```python
from build123d import *

# Parameters (mm, degrees)
F1_DEPTH = 2.2
F3_DEPTH = 3


with BuildPart() as f1:
    # F0 (on Front) → F1 (new body)
    with BuildSketch(Plane.XZ):
        with BuildLine():
            Line((12.5, -9.5), (12.5, 9.5))
            Line((12.5, 9.5), (3.2765988609, 9.5))
            Line((3.2765988609, 9.5), (3.2765988609, 0.1127291822))
            ThreePointArc((3.2765988609, 0.1127291822), (0.0399120355, -3.3998448003), (-3.3149907831, 0))
            Line((-3.3149907831, 0), (-3.3149907831, 9.5))
            Line((-3.3149907831, 9.5), (-12.5, 9.5))
            Line((-12.5, 9.5), (-12.5, -9.5))
            Line((-12.5, -9.5), (12.5, -9.5))
        make_face()
    extrude(amount=F1_DEPTH)

    # F2 (on face) → F3 (join)
    with BuildSketch(Plane.XZ.offset(2.2)):
        with BuildLine():
            ThreePointArc((4.6765988609, 0.1539773139), (0.0605272986, -4.799695782), (-4.7154452944, 0))
            Line((-4.7154452944, 0), (-4.7154452944, 9.5))
            Line((-4.7154452944, 9.5), (-12.5, 9.5))
            Line((-12.5, 9.5), (-12.5, -9.5))
            Line((-12.5, -9.5), (12.5, -9.5))
            Line((12.5, -9.5), (12.5, 9.5))
            Line((12.5, 9.5), (4.6765988609, 9.5))
            Line((4.6765988609, 9.5), (4.6765988609, 0.1539773139))
        make_face()
    extrude(amount=F3_DEPTH)


solid = f1.part
```
The model under review builds one solid part; all positions refer to its coordinate system, in mm. A direction names the side the tool comes from. Round coordinates to 2 decimals unless told otherwise and drop trailing zeros. Write each loop counter-clockwise with the first axis right and the second up, starting at its lowest first coordinate (ties: lowest second). Pieces come first, ordered by that corner, then holes. Notation, with made-up numbers: (59, 76) - (99, 76) arc R19 ccw to (99, 106) - close; hole circle Ø2 at (-10, 28). An arc over 180 degrees is marked (long way). One line per question, with ' | ' between items.
Item 1: The part is to be moulded in two halves that separate along X. For faces 1 (the face through (0, -3, -9.5)), 2 (the face through (-12.5, -3, 0)), 3 (the face through (4.677, -4, 5)), 4 (the face through (-4, -2.2, 1)), say which applies: pulls with the +X half, pulls with the -X half, needs draft (parallel to the pull), parting line crosses it, or undercut.
Resolved:
face 1: needs draft | face 2: pulls with the -X half | face 3: undercut | face 4: undercut
Item 2: Add section C-C, the plane z = -0.75. Give the boundary of the cut face in (x, y).
Resolved:
outline: (-12.5, -5.2) - (-4.67, -5.2) - (-4.67, -2.2) - (-3.25, -2.2) - (-3.25, 0) - (-12.5, 0) - close; (3.22, -2.2) - (4.64, -2.2) - (4.64, -5.2) - (12.5, -5.2) - (12.5, 0) - (3.22, 0) - close
Item 3: To check wall thickness, follow probe 1 along X at (y, z) = (-1.7, 0) (3 decimals); probe 2 along X at (y, z) = (-3.2, 4.25); probe 3 along Y at (x, z) = (-3.75, 4.5). State the ranges of each line that lie inside material, in increasing order.
Resolved:
probe 1: x = -12.5 to -3.315, 3.282 to 12.5 | probe 2: x = -12.5 to -4.72, 4.68 to 12.5 | probe 3: y = -2.2 to 0
Item 4: Add section D-D, the plane y = -3.55. Give the boundary of the cut face in (x, z), then the cut area to 3 significant figures.
Resolved:
outline: (-12.5, -9.5) - (12.5, -9.5) - (12.5, 9.5) - (4.68, 9.5) - (4.68, 0.15) arc R4.7 cw (long way) to (-4.72, 0) - (-4.72, 9.5) - (-12.5, 9.5) - close | area: 350 mm2
Item 5: Add section B-B, the plane y = -1.5. Give the boundary of the cut face in (x, z) (3 decimals).
Resolved:
outline: (-12.5, -9.5) - (12.5, -9.5) - (12.5, 9.5) - (3.277, 9.5) - (3.277, 0.113) arc R3.3 cw (long way) to (-3.315, 0) - (-3.315, 9.5) - (-12.5, 9.5) - close
Item 6: For faces 5 (the face through (-4.715, -4, 5)), 6 (the face through (8, -3, 9.5)), 7 (the face through (-3.315, -1, 5)), list the 3-axis set-ups (+Z, -Z, +X, -X, +Y, -Y) from which the entire face can be reached by the end or side of a thin tool; tool diameter is ignored.
Resolved:
face 5: +Z, -Y | face 6: +Z, +X, -X, +Y, -Y | face 7: +Z, +Y, -Y
Item 7: Add section A-A, the plane z = 3. Give the boundary of the cut face in (x, y) (3 decimals), then the cut area to 3 significant figures.
Resolved:
outline: (-12.5, -5.2) - (-4.715, -5.2) - (-4.715, -2.2) - (-3.315, -2.2) - (-3.315, 0) - (-12.5, 0) - close; (3.277, -2.2) - (4.677, -2.2) - (4.677, -5.2) - (12.5, -5.2) - (12.5, 0) - (3.277, 0) - close | area: 87.3 mm2
